The listing builds one solid part. Answer for the finished solid, in the listing's coordinates (mm). Face numbers are marked on the shaded views. A direction names the side the tool comes from. Give positions to 0.01 mm unless a question says otherwise; leave off trailing zeros. Write each loop counter-clockwise with the first axis right and the second up, starting at its lowest first coordinate (ties: lowest second). Pieces come first, ordered by that corner, then holes. Notation, with made-up numbers: (66.25, 9.25) - (92.25, 9.25) arc R30 ccw to (92.25, 45.25) - close; hole circle Ø3 at (35.5, -33.5). An arc over 180 degrees is marked (long way). Answer as CSV lines item,"result". Start each with the question number.
(1) Find section D-D (y = -6). Write down the section's boundary in (x, z).
(2) For a pull along Y with two mould halves and no side action, classify the marked faces 3, 4 and 5 as pulls with the +Y half, pulls with the -Y half, needs draft (parallel to the pull), parting line crosses it, or undercut.
(3) Find section B-B (x = 0). Write down the section's boundary in (y, z), then the cut area to 3 significant figures.
(4) Straight lines are drawn through the part: probe 1 along Y at (x, z) = (0, 0.5); probe 2 along X at (y, z) = (-19, -1.25); probe 3 along Y at (x, z) = (-1.5, 3). For each, find the intervals that lie inside material, in ascending order.
(5) Each of these flat-tipped pins is pushed along its axis until it touches: pin 1 Ø1.5 at (x, y) = (1.5, -10) entering from +Z; pin 2 Ø2.5 at (x, y) = (0, -19) entering from -Z. Where does it stop, or does it pass through?
(6) For the marked faces 1 and 2, determine the directions among +Z, -Z, +X, -X, +Y, -Y from which every point of the face is accessible in a straight line to the end or side of a thin tool.
(7) Find section A-A (y = -19). Write down the section's boundary in (x, z).
(8) Find section C-C (z = -1). Write down the section's boundary in (x, y), then the cut area to 3 significant figures.
from build123d import *

# Parameters (mm, degrees)
SKETCH003_W         = 17
SKETCH003_H         = 8
PAD001_DEPTH        = 24
SKETCH005_R         = 5.15
POCKET_DEPTH        = 7
HOLE002_D           = 3
HOLE002_DEPTH       = 25
HOLE002_CSINK_D     = 6.1
HOLE002_CSINK_ANGLE = 90


with BuildPart() as part:
    # Sketch003 → Pad001 (new body)
    with BuildSketch(Plane.XZ):
        Rectangle(SKETCH003_W, SKETCH003_H)
    extrude(amount=PAD001_DEPTH)

    # Sketch005 → Pocket (cut)
    with BuildSketch(Plane(origin=(0, 0, 4), x_dir=(-1, 0, 0), z_dir=(0, 0, 1))):
        with Locations((0, 6)):
            Circle(SKETCH005_R)
    extrude(amount=-POCKET_DEPTH, mode=Mode.SUBTRACT)

    # Hole002
    with Locations(Plane(origin=(0, 0, 4), x_dir=(-1, 0, 0), z_dir=(0, 0, 1))):
        with Locations((0, 19)):
            CounterSinkHole(HOLE002_D / 2, HOLE002_CSINK_D / 2, depth=HOLE002_DEPTH, counter_sink_angle=HOLE002_CSINK_ANGLE)


solid = part.part
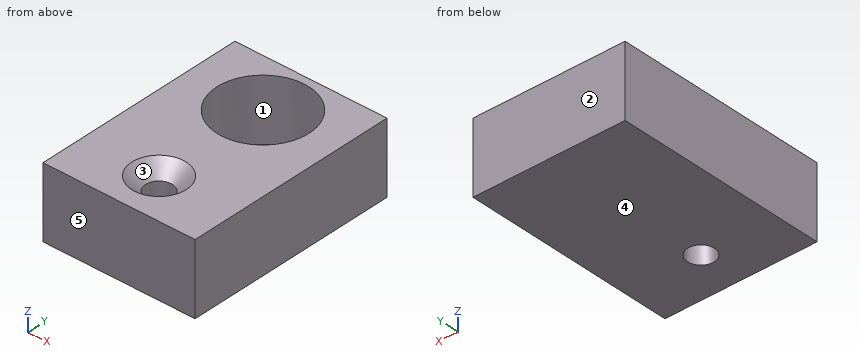
Result set:
1,outline,"(-8.5, -4) - (8.5, -4) - (8.5, 4) - (5.15, 4) - (5.15, -3) - (-5.15, -3) - (-5.15, 4) - (-8.5, 4) - close"
2,face 3,"undercut"
2,face 4,"needs draft"
2,face 5,"pulls with the -Y half"
3,outline,"(-24, -4) - (-20.5, -4) - (-20.5, 2.45) - (-22.05, 4) - (-24, 4) - close; (-17.5, -4) - (0, -4) - (0, 4) - (-0.85, 4) - (-0.85, -3) - (-11.15, -3) - (-11.15, 4) - (-15.95, 4) - (-17.5, 2.45) - close"
3,area,"93.5 mm^2"
4,probe 1,"-24 to -20.5, -17.5 to -11.15, -0.85 to 0"
4,probe 2,"-8.5 to -1.5, 1.5 to 8.5"
4,probe 3,"-24 to -20.4, -17.6 to -10.93, -1.07 to 0"
5,pin 1,"z = -3"
5,pin 2,"through"
6,face 1,"+Z"
6,face 2,"+Z, -Z, +X, -X, +Y"
7,outline,"(-8.5, -4) - (-1.5, -4) - (-1.5, 2.45) - (-3.05, 4) - (-8.5, 4) - close; (1.5, -4) - (8.5, -4) - (8.5, 4) - (3.05, 4) - (1.5, 2.45) - close"
8,outline,"(-8.5, -24) - (8.5, -24) - (8.5, 0) - (-8.5, 0) - close; hole circle Ø10.3 at (0, -6); hole circle Ø3 at (0, -19)"
8,area,"318 mm^2"
